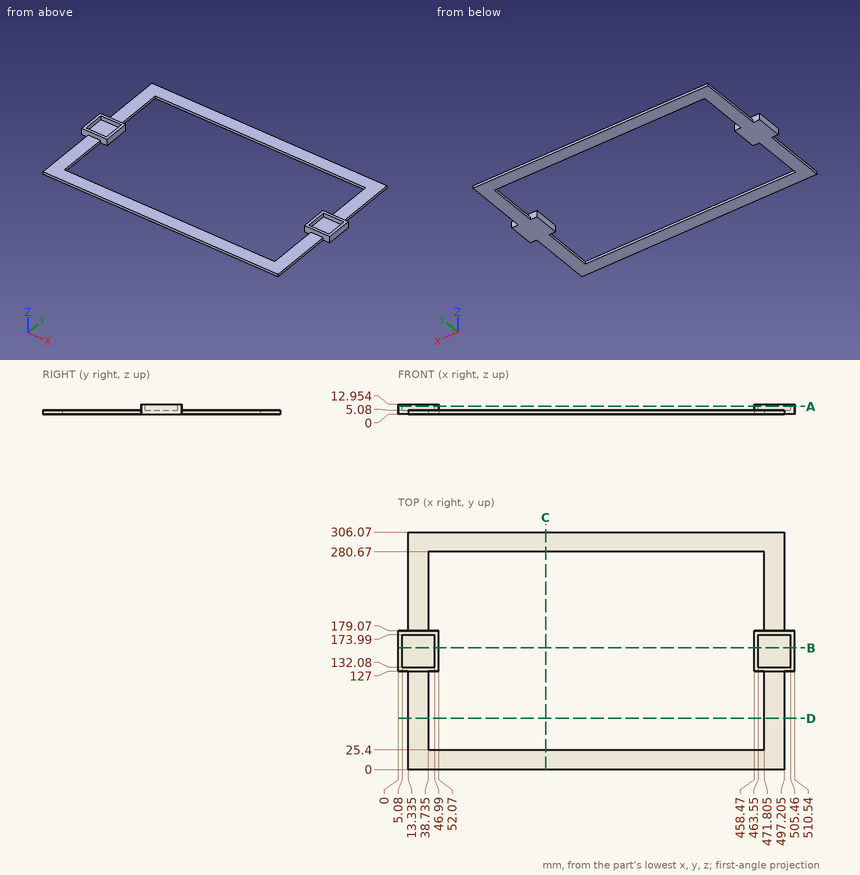
Can you work these out from the drawing? Everything is in mm from the part's minimum corner. Give positions to 0.01 mm unless a question says otherwise; leave off trailing zeros. Order: outer loops, then holes, each group sorted by start corner. A loop starts at its lowest first (then second) coordinate and runs counter-clockwise, first axis right, second up.
1. Suppose I cut it at C-C (x = 190). List the corners of the cut face in (y, z) for me, plus the area to 3 significant figures.
2. I need wall thicknesses on L1, parallel to X at y = 153, z = 3.5; L2, parallel to Y at x = 472, z = 11.25; L3, parallel to Y at x = 263, z = 3. Which ranges of each line are inside material? Lowest first, please.
3. Suppose I cut it at D-D (y = 66). List the corners of the cut face in (x, z) for me (3 decimals), plus the area to 3 significant figures.
4. Suppose I cut it at B-B (y = 157). List the corners of the cut face in (x, z) for me, plus the area to 3 significant figures.
5. Will these pins go through, and if not, where does the flat tip stop? P1, Ø2.5, axis at y = 154, z = 7.5, coming from the -X side; P2, Ø2.5, axis at y = 92.5, z = 1.5, coming from the +X side (3 decimals); P3, Ø2.5, axis at y = 270.5, z = 2, coming from the -X side (3 decimals).
6. Suppose I cut it at A-A (z = 10). List the corners of the cut face in (x, y) for me, plus the area to 3 significant figures.
Solved:
1. outline: (0, 0) - (25.4, 0) - (25.4, 5.08) - (0, 5.08) - close; (280.67, 0) - (306.07, 0) - (306.07, 5.08) - (280.67, 5.08) - close
1. area: 258 mm2
2. L1: x = 0 to 52.07, 458.47 to 510.54
2. L2: y = 127 to 132.08, 173.99 to 179.07
2. L3: y = 0 to 25.4, 280.67 to 306.07
3. outline: (13.335, 0) - (38.735, 0) - (38.735, 5.08) - (13.335, 5.08) - close; (471.805, 0) - (497.205, 0) - (497.205, 5.08) - (471.805, 5.08) - close
3. area: 258 mm2
4. outline: (0, 0) - (52.07, 0) - (52.07, 12.95) - (46.99, 12.95) - (46.99, 5.08) - (5.08, 5.08) - (5.08, 12.95) - (0, 12.95) - close; (458.47, 0) - (510.54, 0) - (510.54, 12.95) - (505.46, 12.95) - (505.46, 5.08) - (463.55, 5.08) - (463.55, 12.95) - (458.47, 12.95) - close
4. area: 689 mm2
5. P1: stops at x = 0
5. P2: stops at x = 497.205
5. P3: stops at x = 13.335
6. outline: (0, 127) - (52.07, 127) - (52.07, 179.07) - (0, 179.07) - close; (458.47, 127) - (510.54, 127) - (510.54, 179.07) - (458.47, 179.07) - close; hole (5.08, 132.08) - (46.99, 132.08) - (46.99, 173.99) - (5.08, 173.99) - close; hole (463.55, 132.08) - (505.46, 132.08) - (505.46, 173.99) - (463.55, 173.99) - close
6. area: 1,910 mm2
